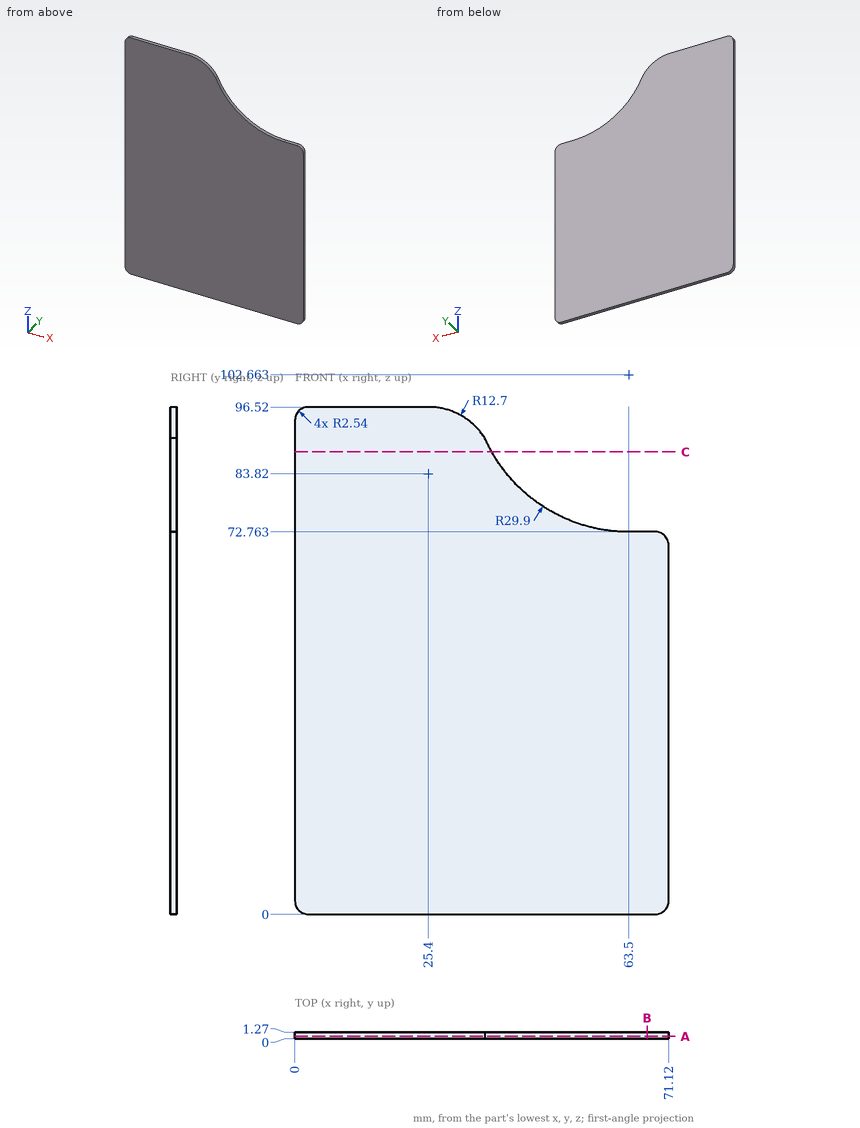
Geometry check sheet. Reference: drawing and pictorial views, mm from the part's lowest x, y, z. Give positions to 0.01 mm unless a question says otherwise; leave off trailing zeros. Order: outer loops, then holes, each group sorted by start corner. A loop starts at its lowest first (then second) coordinate and runs counter-clockwise, first axis right, second up. Notation, with made-up numbers: M -14.75,31.5 L 19.25,31.5 A34 ccw 19.25,62.5 Z; hole C 83,46 d4. An arc over 180 degrees is marked long. Answer in a Markdown table with one row per item. Add a question column.
Q1. Sectioned sample at C-C, the plane z = 88. Record the boundary of the cut face in (x, y).
Q2. Sectioned sample at B-B, the plane x = 67. Record the boundary of the cut face in (y, z).
Q3. Thickness scan on L1, parallel to Z at x = 49, y = 0.8 (1 decimal); L2, parallel to X at y = 0.6, z = 92.5; L3, parallel to X at y = 0.5, z = 83 (1 decimal). Record the ranges inside material, lowest first.
Q4. Sectioned sample at A-A, the plane y = 0.5. Record the boundary of the cut face in (x, z) (1 decimal), and give its area (3 significant figures).
Verdict:
| question | item | result |
|---|---|---|
| 1 | outline | M 0,0 L 37.44,0 L 37.44,1.27 L 0,1.27 Z |
| 2 | outline | M 0,0 L 1.27,0 L 1.27,72.76 L 0,72.76 Z |
| 3 | L1 | 0 to 76.5 |
| 3 | L2 | 0 to 34.67 |
| 3 | L3 | 0 to 41 |
| 4 | outline | M 0,2.5 A2.5 ccw 2.5,0 L 68.6,0 A2.5 ccw 71.1,2.5 L 71.1,70.2 A2.5 ccw 68.6,72.8 L 63.5,72.8 A29.9 cw 36.1,90.6 A12.7 ccw 25.4,96.5 L 2.5,96.5 A2.5 ccw 0,94 Z |
| 4 | area | 6,150 mm² |
